Build history of the part. All positions in model axes, mm. A direction names the side the tool comes from. Coordinates: 2 decimals unless noted, no trailing zeros. Loops run counter-clockwise (first coordinate to the right, second up) from the corner with the lowest first, then second, coordinate; pieces in that order, holes last.
Item 1: Flat gauge pin, fed straight in: pin 1 (16 mm diameter, centred on y = 134.5, z = 21, fed in from -X). Where does the tip first touch, or does it go through?
Item 2: Cut at B-B (x = 41.5). List the corners of the cut face in (y, z), and give its area (3 significant figures).
Item 3: 3-axis set-ups, long thin cutter, end or side, ignore diameter. For faces 1 (the face through (15.66, 105.957, 15.715)), 2 (the face through (102, 203.2, 25)): which of +Z, -Z, +X, -X, +Y, -Y reach the whole face in a straight line?
Item 4: Cut at C-C (y = 145). List the corners of the cut face in (x, z), and give its area (3 significant figures).
Item 5: Cut at A-A (z = 18). List the corners of the cut face in (x, y), and give its area (3 significant figures).
Item 6: Drill centre lines: line 1 along X through (y, z) = (54.5, 21); line 2 along Y through (x, z) = (162.5, 12.5); line 3 along Y through (x, z) = (35, 22). Where is each one in solid material? Low to high.
from build123d import *

# Parameters (mm, degrees)
BOSS_EXTRUDE1_DEPTH = 49.784
CUT_EXTRUDE1_DEPTH  = 31.877


with BuildPart() as part:
    # Sketch1 → Boss-Extrude1 (new body)
    with BuildSketch(Plane.XY):
        Polygon((0, 199.644), (3.556, 203.2), (202.7936, 203.2), (206.3496, 199.644), (206.3496, 3.556), (202.7936, 0), (3.556, 0), (0, 3.556), align=None)
    extrude(amount=BOSS_EXTRUDE1_DEPTH)

    # Sketch2 → Cut-Extrude1 (cut)
    with BuildSketch(Plane(origin=(0, 0, 0), x_dir=(-1, 0, 0), z_dir=(0, 0, -1))):
        with BuildLine():
            Line((-192.8876, 181.8386), (-192.8876, 21.3614))
            ThreePointArc((-192.8876, 21.3614), (-190.49952443, 15.59607557), (-184.7342, 13.208))
            Line((-184.7342, 13.208), (-65.913, 13.208))
            ThreePointArc((-65.913, 13.208), (-60.14767557, 15.59607557), (-57.7596, 21.3614))
            Line((-57.7596, 21.3614), (-57.7596, 100.076))
            Line((-57.7596, 100.076), (-54.2036, 103.632))
            Line((-54.2036, 103.632), (-21.3614, 103.632))
            ThreePointArc((-21.3614, 103.632), (-15.59607557, 106.02007557), (-13.208, 111.7854))
            Line((-13.208, 111.7854), (-13.208, 181.8386))
            ThreePointArc((-13.208, 181.8386), (-15.59607557, 187.60392443), (-21.3614, 189.992))
            Line((-21.3614, 189.992), (-184.7342, 189.992))
            ThreePointArc((-184.7342, 189.992), (-190.49952443, 187.60392443), (-192.8876, 181.8386))
        make_face()
    extrude(amount=-CUT_EXTRUDE1_DEPTH, mode=Mode.SUBTRACT)


solid = part.part
Filled sheet:
1. pin 1: stops at x = 0
2. outline: (0, 0) - (103.63, 0) - (103.63, 31.88) - (189.99, 31.88) - (189.99, 0) - (203.2, 0) - (203.2, 49.78) - (0, 49.78) - close
2. area: 7,360 mm2
3. face 1: -Z
3. face 2: +Z, -Z, +X, -X, +Y
4. outline: (0, 0) - (13.21, 0) - (13.21, 31.88) - (192.89, 31.88) - (192.89, 0) - (206.35, 0) - (206.35, 49.78) - (0, 49.78) - close
4. area: 4,550 mm2
5. outline: (0, 3.56) - (3.56, 0) - (202.79, 0) - (206.35, 3.56) - (206.35, 199.64) - (202.79, 203.2) - (3.56, 203.2) - (0, 199.64) - close; hole (13.21, 111.79) arc R8.15 ccw to (21.36, 103.63) - (54.2, 103.63) - (57.76, 100.08) - (57.76, 21.36) arc R8.15 ccw to (65.91, 13.21) - (184.73, 13.21) arc R8.15 ccw to (192.89, 21.36) - (192.89, 181.84) arc R8.15 ccw to (184.73, 189.99) - (21.36, 189.99) arc R8.15 ccw to (13.21, 181.84) - close
5. area: 14,200 mm2
6. line 1: x = 0 to 57.76, 192.89 to 206.35
6. line 2: y = 0 to 13.21, 189.99 to 203.2
6. line 3: y = 0 to 103.63, 189.99 to 203.2
